For this review, use the dimensioned drawing (mm, ordinates from the lowest corner) and the shaded views. Give positions to 0.01 mm unless a question says otherwise; leave off trailing zeros. Write each loop counter-clockwise with the first axis right and the second up, starting at its lowest first coordinate (ties: lowest second). Pieces come first, ordered by that corner, then holes. Notation, with made-up numbers: (-14.5, 62.5) -> (-0.5, 62.5) arc R22 cw to (-0.5, 96.5) -> close; hole circle Ø11 at (7.5, 84). An arc over 180 degrees is marked (long way). Return JSON: item names as keys, results as strings.
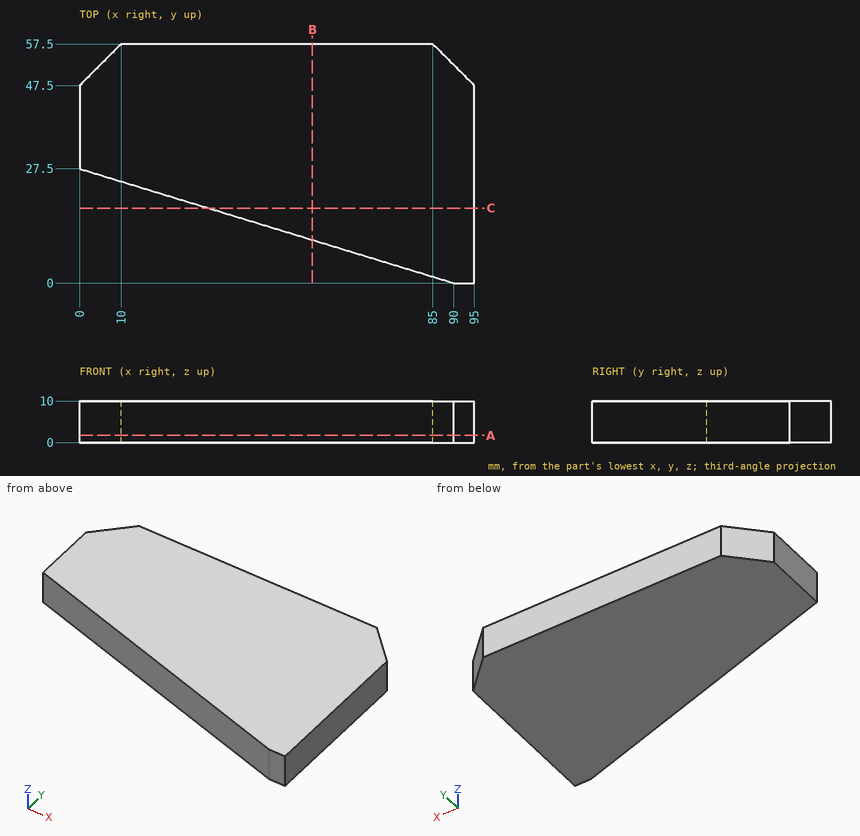
1. Add section C-C, the plane y = 18. State the section outline as (x, z) points.
Results found:
{"outline": "(31.09, 0) -> (95, 0) -> (95, 10) -> (31.09, 10) -> close"}
2. Add section B-B, the plane x = 56. State the section outline as (y, z) points, plus the area to 3 significant figures.
Results found:
{"outline": "(10.39, 0) -> (57.5, 0) -> (57.5, 10) -> (10.39, 10) -> close", "area": "471 mm²"}
3. For pin 1 (3 mm diameter, centred on x = 16.5, z = 3.5, fed in from -Y); pin 2 (2 mm diameter, centred on y = 48, z = 7.5, fed in from +X), all flat-tipped, find the tip position at first contact; note any pin that passes through.
Results found:
{"pin 1": "stops at y = 22", "pin 2": "stops at x = 95"}
4. To check wall thickness, follow probe 1 along X at (y, z) = (50, 2.5); probe 2 along Y at (x, z) = (88, 6); probe 3 along Y at (x, z) = (33, 9.25). State the ranges of each line that lie inside material, in increasing order.
Results found:
{"probe 1": "x = 2.5 to 92.5", "probe 2": "y = 0.61 to 54.5", "probe 3": "y = 17.42 to 57.5"}
5. Add section A-A, the plane z = 1.75. State the section outline as (x, y) points.
Results found:
{"outline": "(0, 27.5) -> (90, 0) -> (95, 0) -> (95, 47.5) -> (85, 57.5) -> (10, 57.5) -> (0, 47.5) -> close"}
